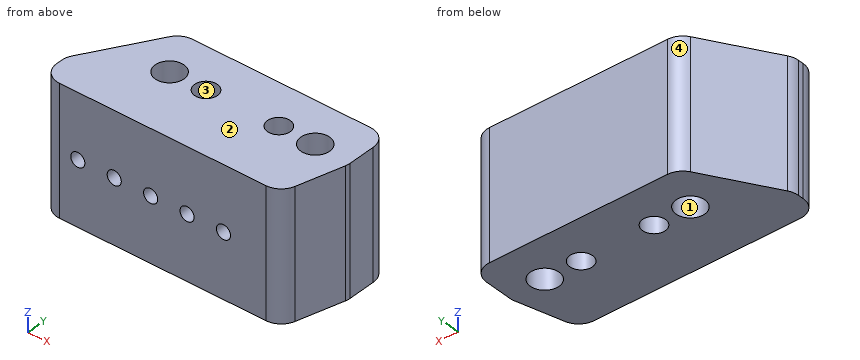
Autodesk Inventor part; units mm, degrees
ref_plane "YZ Plane" through (0, 0, 0) normal (1, 0, 0) x (0, 1, 0)
ref_plane "XZ Plane" through (0, 0, 0) normal (0, 1, 0) x (-1, 0, 0)
ref_plane "XY Plane" through (0, 0, 0) normal (0, 0, 1) x (1, 0, 0)
sketch "Sketch1" plane through (0, 0, 0) normal (0, 0, 1) x (1, 0, 0)
  line L0 (19.05, 7.62) -> (-25.4, 7.62)
  line L1 (-25.4, 7.62) -> (-25.4, -11.43)
  line L2 (-25.4, -11.43) -> (19.05, -11.43)
  line L3 (19.05, -11.43) -> (19.05, 7.62)
  line L4 (19.05, 7.62) -> (-25.4, -11.43) construction
  line L5 (-25.4, 7.62) -> (19.05, -11.43) construction
  line L6 (0, 11.43) -> (0, -15.24) construction
  line L7 (-34.29, 0) -> (27.94, 0) construction
  point P0 (-3.175, -1.905)
  dimension "d0" = 19.05
  dimension "d1" = 44.45
  dimension "d56" = 25.4
  dimension "d93" = 11.43
extrude "Extrusion1" add sketch "Sketch1" along normal mid plane 22.225
sketch "Sketch3" plane through (0, 0, 11.1125) normal (0, 0, 1) x (1, 0, 0)
  line L0 (-12.7, 0) -> (12.7, 0) construction
  point P0 (0, 0)
  point P1 (0, 0)
  dimension "d35" = 25.4
hole "Hole1" at (-12.7, 0, 11.1125) at (12.7, 0, 11.1125) direction (0, 0, -1) diameter 5.0038 end through all
sketch "Sketch4" plane through (0, 0, 11.1125) normal (0, 0, 1) x (1, 0, 0)
  line L0 (-6.35, 0) -> (6.35, 0) construction
  point P0 (0, 0)
  point P1 (0, 0)
  dimension "d43" = 12.7
hole "Hole2" at (-6.35, 0, 11.1125) at (6.35, 0, 11.1125) direction (0, 0, -1) diameter 3.9624 end through all
sketch "Sketch6" plane through (-25.4, -11.43, 11.1125) normal (0, -1, 0) x (1, 0, 0)
  line L0 (25.4, -11.1125) -> (6.35, -11.1125) construction
  point P0 (12.7, -11.1125)
  point P1 (12.7, -11.1125)
  point P2 (19.05, -11.1125)
  point P3 (19.05, -11.1125)
  point P4 (25.4, -11.1125)
  point P5 (25.4, -11.1125)
  point P6 (31.75, -11.1125)
  point P7 (31.75, -11.1125)
  point P8 (25.4, -11.1125)
  dimension "d83" = 19.05
  dimension "d84" = 6.35
hole "Hole4" at (-19.05, -11.43, 0) at (-12.7, -11.43, 0) at (-6.35, -11.43, 0) at (0, -11.43, 0) at (6.35, -11.43, 0) direction (0, 1, 0) diameter 2.459 depth 8.7884 tip angle 118
chamfer "Chamfer2" distance 10.668 angle 15 1 edges at (19.05, -11.43, 0) measured on face at (19.05, -5.08, -3.7042)
chamfer "Chamfer3" distance 13.97 angle 31.215 1 edges at (-25.4, 7.62, 0) measured on face at (-25.4, -5.08, 3.7042)
fillet "Fillet1" radius 3.175 6 edges at (16.1915, -11.43, 0) (-25.4, -11.43, 0) (-25.4, -6.35, 0) (-16.9346, 7.62, 0) (19.05, 7.62, 0) (19.05, -0.762, 0)
properties part number "BRACE,CHAIN,#25,ELEVATOR" material "Aluminum 7075"
The listing builds one solid part. Answer for the finished solid, in the listing's coordinates (mm). Face numbers are marked on the shaded views. Coordinates: 2 decimals unless noted, no trailing zeros. Order: outer loops, then holes, each group sorted by start corner. A loop starts at its lowest first (then second) coordinate and runs counter-clockwise, first axis right, second up. Notation, with made-up numbers: M -29.5,82.25 L 0.5,82.25 A12 ccw 0.5,86.25 Z; hole C -9,38.25 d5. An arc over 180 degrees is marked long. Answer as a JSON object with one key per item and string values. Group by question number.
1. Straight lines are drawn through the part: line 1 (X direction, y = 0, z = -2.75); line 2 (X direction, y = -0.5, z = 0.75); line 3 (Y direction, x = 12.5, z = 0.5). For each, find the intervals that lie inside material, in ascending order.
2. Section C-C on y = 1.5 is taken. Write down the section's boundary in (x, z), then the cut area to 3 significant figures.
3. Determine the mould class of the marked faces 1, 2, 3 and 4 for opening direction Y: released by +Y, released by -Y, zero draft, split by the parting line, or undercut.
4. Section B-B on z = 2.5 is taken. Write down the section's boundary in (x, y) (3 decimals).
5. Flat-ended cylindrical pins translate along their axes: P1, Ø4, axis at y = 3, z = -4, coming from the -X side; P2, Ø2, axis at x = -12.7, z = 0, coming from the -Y side; P3, Ø8, axis at y = -4.5, z = 6, coming from the +X side. Find the tip coordinate at first contact, or state that the pin passes through.
6. Section A-A on x = -12.7 is taken. Write down the section's boundary in (y, z), then the cut area to 3 significant figures.
7. Section D-D on y = 3.5 is taken. Write down the section's boundary in (x, z), then the cut area to 3 significant figures.
Values follow:
{
 "1": {"line 1": "-21.55 to -15.2, -10.2 to -8.33, -4.37 to 4.37, 8.33 to 10.2, 15.2 to 19.05", "line 2": "-21.86 to -15.15, -10.25 to -8.27, -4.43 to 4.43, 8.27 to 10.25, 15.15 to 19.05", "line 3": "-11.43 to -2.49, 2.49 to 7.62"},
 "2": {"outline": "M -20.64,-11.11 L -14.7,-11.11 L -14.7,11.11 L -20.64,11.11 Z; M -10.7,-11.11 L -7.64,-11.11 L -7.64,11.11 L -10.7,11.11 Z; M -5.06,-11.11 L 5.06,-11.11 L 5.06,11.11 L -5.06,11.11 Z; M 7.64,-11.11 L 10.7,-11.11 L 10.7,11.11 L 7.64,11.11 Z; M 14.7,-11.11 L 19.05,-11.11 L 19.05,11.11 L 14.7,11.11 Z", "area": "589 mm2"},
 "3": {"face 1": "undercut", "face 2": "zero draft", "face 3": "undercut", "face 4": "released by +Y"},
 "4": {"outline": "M -25.4,-8.255 A3.175 ccw -22.225,-11.43 L 13.755,-11.43 A3.175 ccw 16.822,-9.077 L 18.942,-1.166 A3.175 ccw 19.05,-0.344 L 19.05,4.445 A3.175 ccw 15.875,7.62 L -15.146,7.62 A3.175 ccw -17.861,6.09 L -24.94,-5.591 A3.175 ccw -25.4,-7.237 Z; hole C -12.7,0 d5.004; hole C -6.35,0 d3.962; hole C 6.35,0 d3.962; hole C 12.7,0 d5.004"},
 "5": {"P1": "x = -20.95", "P2": "y = -2.5", "P3": "x = 19.05"},
 "6": {"outline": "M -11.43,-11.11 L -2.5,-11.11 L -2.5,-1 L -2.64,-1.23 L -11.43,-1.23 Z; M -11.43,1.23 L -2.64,1.23 L -2.5,1 L -2.5,11.11 L -11.43,11.11 Z; M 2.5,-11.11 L 7.62,-11.11 L 7.62,11.11 L 2.5,11.11 Z", "area": "290 mm2"},
 "7": {"outline": "M -19.43,-11.11 L 19.05,-11.11 L 19.05,11.11 L -19.43,11.11 Z", "area": "855 mm2"}
}
